The model under review builds one solid part; all positions refer to its coordinate system, in mm. Coordinates: 2 decimals unless noted, no trailing zeros. Write each loop counter-clockwise with the first axis right and the second up, starting at its lowest first coordinate (ties: lowest second). Pieces come first, ordered by that corner, then holes. Notation, with made-up numbers: (69.5, 40.25) - (107.5, 40.25) arc R15 cw to (107.5, 53.25) - close; hole circle Ø5 at (-40, 70). An arc over 180 degrees is marked (long way). Use one line per item in the form item = value. Start each with the question number.
```python
from build123d import *

# Parameters (mm, degrees)
F0_W     = 430
F0_H     = 40
F0_R     = 3
F1_DEPTH = 19
F2_R     = 19.99999
F3_R     = 3
F4_DEPTH = 19.001


# Not quite as in the source:
# - a fillet or chamfer is up to 0.001 mm smaller than in the source, because OpenCascade refuses the exact size


with BuildPart() as f1:
    # F0 (on Right) → F1 (new body)
    with BuildSketch(Plane.YZ):
        with Locations((-200, 0)):
            Rectangle(F0_W, F0_H)
        with Locations((-400, 0)):
            Circle(F0_R, mode=Mode.SUBTRACT)
        Circle(F0_R, mode=Mode.SUBTRACT)
    extrude(amount=F1_DEPTH)

    # F2 (radius 20 in the source; OpenCascade refuses exactly that, so slightly less here)
    f2_edges = [f1.edges().sort_by_distance(p)[0] for p in [
        (9.5, 15, 20),
        (9.5, 15, -20),
        (9.5, -415, 20),
        (9.5, -415, -20),
    ]]
    fillet(f2_edges, radius=F2_R)

    # F3 (on face) → F4 (cut, through all)
    with BuildSketch(Plane.YZ.offset(19)):
        with Locations((-300, 0)):
            Circle(F3_R)
    extrude(amount=-F4_DEPTH, mode=Mode.SUBTRACT)


solid = f1.part
```
1. For L1, parallel to Z at x = 9.5, y = 0; L2, parallel to Y at x = 12.5, z = -6; L3, parallel to Y at x = 6, z = -8, list the stretches that pass through material, from the lowest coordinate up.
2. Take a section at B-B (z = 13). State the section outline as (x, y) points.
3. For P1, Ø6, axis at x = 8.5, z = -7.5, coming from the +Y side; P2, Ø8, axis at y = -400, z = 0, coming from the +X side; P3, Ø2, axis at x = 9.5, z = 14.5, coming from the -Y side; P4, Ø6, axis at x = 5, z = 7, coming from the +Y side, all flat-tipped, find the tip position at first contact; note any pin that passes through.
4. Take a section at A-A (x = 5.5). Count the separate pieces of the cut face and the enclosed holes in it, plus the area to 3 significant figures.
Returned:
q1.L1 = -19.36 to -3, 3 to 19.36
q1.L2 = -414.08 to 14.08
q1.L3 = -413.33 to 13.33
q2.outline = (0, -410.2) - (19, -410.2) - (19, 10.2) - (0, 10.2) - close
q3.P1 = 14.49
q3.P2 = 19
q3.P3 = -409.76
q3.P4 = 14.6
q4.separate_pieces = 1
q4.enclosed_holes = 3
q4.area = 16,800 mm²
